Verification items for the finished model (mm, model axes). Round coordinates to 2 decimals unless told otherwise and drop trailing zeros. Order: outer loops, then holes, each group sorted by start corner. A loop starts at its lowest first (then second) coordinate and runs counter-clockwise, first axis right, second up. Notation, with made-up numbers: (0.5, -30.5) -> (38.5, -30.5) arc R24 cw to (38.5, -19.5) -> close; hole circle Ø3 at (-8.75, 85.5). An arc over 180 degrees is marked (long way). Return JSON: item names as keys, results as strings. Group by question number.
Item 1: Draft check along Y on faces 1 (the flat face through (3, 0, 0)), 2 (the cylindrical face through (-0.325, -10.464, 3.549)), 3 (the conical face through (11.443, 3.604, 6.66)). Enter one of: pulls with the +Y half, pulls with the -Y half, needs draft (parallel to the pull), parting line crosses it, or undercut.
Item 2: Scan lines: probe 1 along Y at (x, z) = (8.5, 3.75); probe 2 along Y at (x, z) = (-1.25, 5.5); probe 3 along Y at (x, z) = (7.25, 1.5). Record each from-to range of solid material in increasing order. Write a range as from..to.
Item 3: Sectioned sample at A-A on y = 0. Record the cut outline in (x, z) (3 decimals), plus the area to 3 significant figures.
Item 4: Depth check by flat-ended pin: pin 1 Ø4 at (x, z) = (3, 1.5) entering from -Y; pin 2 Ø3 at (x, z) = (-6, 2) entering from -Y; pin 3 Ø1.5 at (y, z) = (10, 1) entering from +X. Enter the tip coordinate at first touch or a pass-through.
Item 5: Sectioned sample at D-D on z = 1.5. Record the cut outline in (x, y) (3 decimals).
Item 6: Sectioned sample at B-B on x = 0. Record the cut outline in (y, z) (3 decimals).
Item 7: Sectioned sample at C-C on z = 5.25. Record the cut outline in (x, y) (3 decimals).
```python
from build123d import *

# Parameters (mm, degrees)
SKETCH1_R           = 13.9
BOSS_EXTRUDE1_DEPTH = 7
CUT_EXTRUDE1_REACH  = 22.867
SKETCH2_R           = 1.585
CUT_EXTRUDE2_REACH  = 22.867
SKETCH3_R           = 1.5
CHAMFER1_SIZE       = 7
CHAMFER1_SIZE_2     = 2


with BuildPart() as part:
    # Sketch1 → Boss-Extrude1 (new body)
    with BuildSketch(Plane.XY):
        Circle(SKETCH1_R)
    extrude(amount=BOSS_EXTRUDE1_DEPTH)

    # Sketch2 → Cut-Extrude1 (cut, up to next)
    with BuildSketch(Plane.XY.offset(7), mode=Mode.PRIVATE) as cut_extrude1_sk1:
        Circle(SKETCH2_R)
    cut_extrude1_tool1 = extrude(cut_extrude1_sk1.sketch, amount=-CUT_EXTRUDE1_REACH, mode=Mode.PRIVATE) & part.part
    add(cut_extrude1_tool1.solids().sort_by_distance((0, 0, 7))[0], mode=Mode.SUBTRACT)

    # Sketch3 → Cut-Extrude2 (cut, up to next)
    with BuildSketch(Plane.XY.offset(7), mode=Mode.PRIVATE) as cut_extrude2_sk1:
        with Locations((-8, 0)):
            Circle(SKETCH3_R)
    cut_extrude2_tool1 = extrude(cut_extrude2_sk1.sketch, amount=-CUT_EXTRUDE2_REACH, mode=Mode.PRIVATE) & part.part
    # Sketch3 → Cut-Extrude2 (cut, up to next)
    with BuildSketch(Plane.XY.offset(7), mode=Mode.PRIVATE) as cut_extrude2_sk2:
        with Locations((8, 0)):
            Circle(SKETCH3_R)
    cut_extrude2_tool2 = extrude(cut_extrude2_sk2.sketch, amount=-CUT_EXTRUDE2_REACH, mode=Mode.PRIVATE) & part.part
    # Sketch3 → Cut-Extrude2 (cut, up to next)
    with BuildSketch(Plane.XY.offset(7), mode=Mode.PRIVATE) as cut_extrude2_sk3:
        with Locations((0, -9)):
            Circle(SKETCH3_R)
    cut_extrude2_tool3 = extrude(cut_extrude2_sk3.sketch, amount=-CUT_EXTRUDE2_REACH, mode=Mode.PRIVATE) & part.part
    # Sketch3 → Cut-Extrude2 (cut, up to next)
    with BuildSketch(Plane.XY.offset(7), mode=Mode.PRIVATE) as cut_extrude2_sk4:
        with Locations((0, 9)):
            Circle(SKETCH3_R)
    cut_extrude2_tool4 = extrude(cut_extrude2_sk4.sketch, amount=-CUT_EXTRUDE2_REACH, mode=Mode.PRIVATE) & part.part
    add(cut_extrude2_tool1.solids().sort_by_distance((-8, 0, 7))[0], mode=Mode.SUBTRACT)
    add(cut_extrude2_tool2.solids().sort_by_distance((8, 0, 7))[0], mode=Mode.SUBTRACT)
    add(cut_extrude2_tool3.solids().sort_by_distance((0, -9, 7))[0], mode=Mode.SUBTRACT)
    add(cut_extrude2_tool4.solids().sort_by_distance((0, 9, 7))[0], mode=Mode.SUBTRACT)

    # Chamfer1
    # the kernel refuses this chamfer: 7, 2 mm, written as the material it takes off along each edge
    with BuildSketch(Plane(origin=(0, 0, 7), x_dir=(1, 0, 0), z_dir=(0, -1, 0))) as chamfer1_piece_1:
        Polygon((13.9, -CHAMFER1_SIZE), (13.9 - CHAMFER1_SIZE_2, 0), (13.9, 0), align=None)
    revolve(axis=Axis((0, 0, 7), (0, 0, 1)), mode=Mode.SUBTRACT)


solid = part.part
```
Recorded:
{
 "1": {"face 1": "needs draft", "face 2": "undercut", "face 3": "parting line crosses it"},
 "2": {"probe 1": "-9.61..-1.41, 1.41..9.61", "probe 2": "-12.27..-9.83, -8.17..-0.97, 0.97..8.17, 9.83..12.27", "probe 3": "-11.35..-1.3, 1.3..11.35"},
 "3": {"outline": "(-13.9, 0) -> (-9.5, 0) -> (-9.5, 7) -> (-11.9, 7) -> close; (-6.5, 0) -> (-1.585, 0) -> (-1.585, 7) -> (-6.5, 7) -> close; (1.585, 0) -> (6.5, 0) -> (6.5, 7) -> (1.585, 7) -> close; (9.5, 0) -> (13.9, 0) -> (11.9, 7) -> (9.5, 7) -> close", "area": "116 mm²"},
 "4": {"pin 1": "y = -13.8", "pin 2": "y = -12.71", "pin 3": "x = 10.05"},
 "5": {"outline": "circle Ø26.943 at (0, 0); hole circle Ø3 at (-8, 0); hole circle Ø3.17 at (0, 0); hole circle Ø3 at (0, -9); hole circle Ø3 at (0, 9); hole circle Ø3 at (8, 0)"},
 "6": {"outline": "(-13.9, 0) -> (-10.5, 0) -> (-10.5, 7) -> (-11.9, 7) -> close; (-7.5, 0) -> (-1.585, 0) -> (-1.585, 7) -> (-7.5, 7) -> close; (1.585, 0) -> (7.5, 0) -> (7.5, 7) -> (1.585, 7) -> close; (10.5, 0) -> (13.9, 0) -> (11.9, 7) -> (10.5, 7) -> close"},
 "7": {"outline": "circle Ø24.8 at (0, 0); hole circle Ø3 at (-8, 0); hole circle Ø3.17 at (0, 0); hole circle Ø3 at (0, -9); hole circle Ø3 at (0, 9); hole circle Ø3 at (8, 0)"}
}
